Verification items for the finished model (mm, model axes). Face numbers are marked on the shaded views. A direction names the side the tool comes from. Give positions to 0.01 mm unless a question says otherwise; leave off trailing zeros. Write each loop counter-clockwise with the first axis right and the second up, starting at its lowest first coordinate (ties: lowest second). Pieces come first, ordered by that corner, then holes. Notation, with made-up numbers: M -5,35 L 21,35 A7 cw 21,43 Z; hole C -30.5,41.25 d10. An arc over 180 degrees is marked long. Write item = value, one per line.
from build123d import *

# Parameters (mm, degrees)
SKETCH_1_W          = 42
SKETCH_1_H          = 7
SKETCH_1_R          = 1.55
EXTRUDE_5_DEPTH     = 3
SKETCH_1_6_W        = 42
SKETCH_1_6_H        = 2
EXTRUDE_6_DEPTH     = 13
CUT_EXTRUDE_1_DEPTH = 13


with BuildPart() as part:
    # Sketch 1 → Extrude 5 (new body)
    with BuildSketch(Plane.XY):
        with Locations((26, 8.5)):
            Rectangle(SKETCH_1_W, SKETCH_1_H)
        with Locations((12, 8.4)):
            Circle(SKETCH_1_R, mode=Mode.SUBTRACT)
        with Locations((40, 8.4)):
            Circle(SKETCH_1_R, mode=Mode.SUBTRACT)
    extrude(amount=EXTRUDE_5_DEPTH)

    # Sketch 1_6 → Extrude 6 (add)
    with BuildSketch(Plane.XY):
        with Locations((26, 13)):
            Rectangle(SKETCH_1_6_W, SKETCH_1_6_H)
    extrude(amount=EXTRUDE_6_DEPTH)

    # Sketch 4 → Cut-Extrude 1 (cut)
    with BuildSketch(Plane(origin=(0, 14, 0), x_dir=(1, 0, 0), z_dir=(0, 1, 0))):
        with BuildLine():
            ThreePointArc((15, -6.45), (13.45, -8), (15, -9.55))
            Line((15, -9.55), (15, -6.45))
        make_face()
        with BuildLine():
            Line((15, -6.45), (15, -9.55))
            ThreePointArc((15, -9.55), (16.096015511, -9.096015511), (16.55, -8))
            ThreePointArc((16.55, -8), (16.096015511, -6.903984489), (15, -6.45))
        make_face()
        with BuildLine():
            ThreePointArc((37, -6.45), (35.45, -8), (37, -9.55))
            Line((37, -9.55), (37, -6.45))
        make_face()
        with BuildLine():
            Line((37, -6.45), (37, -9.55))
            ThreePointArc((37, -9.55), (38.096015511, -9.096015511), (38.55, -8))
            ThreePointArc((38.55, -8), (38.096015511, -6.903984489), (37, -6.45))
        make_face()
    extrude(amount=-CUT_EXTRUDE_1_DEPTH, mode=Mode.SUBTRACT)


solid = part.part
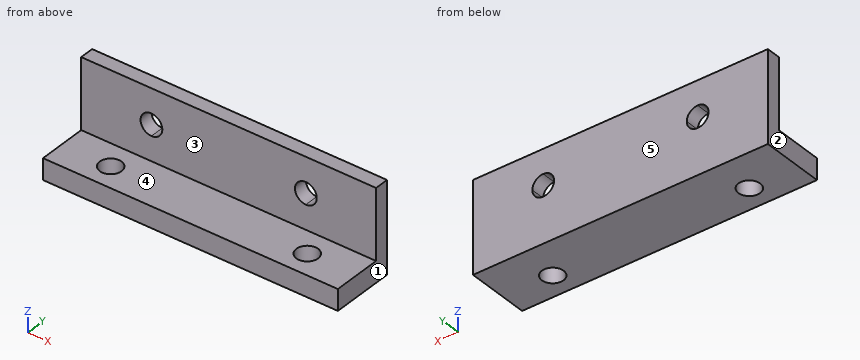
1) Depth check by flat-ended pin: P1, Ø3.5, axis at x = 32, y = 7, coming from the +Z side. Enter the tip coordinate at first touch or a pass-through.
From the geometry:
P1 = 3
2) Cross-section at D-D on x = 30.5. Record the boundary of the cut face in (y, z), plus the area to 3 significant figures.
From the geometry:
outline = M 5,0 L 14,0 L 14,13 L 12,13 L 12,3 L 5,3 Z
area = 47.0 mm^2
3) Tool access check on the marked faces 4 and 5. Record the directions out of +Z, -Z, +X, -X, +Y, -Y that give a thin tool (end or side, any length) a straight path to the whole face; none if there is none.
From the geometry:
face_4 = +Z, +X, -X, -Y
face_5 = +Z, -Z, +X, -X, +Y
4) Cross-section at B-B on y = 8.4. Record the boundary of the cut face in (x, z), plus the area to 3 significant figures.
From the geometry:
outline = M 5,0 L 10.45,0 L 10.45,3 L 5,3 Z; M 13.55,0 L 38.45,0 L 38.45,3 L 13.55,3 Z; M 41.55,0 L 47,0 L 47,3 L 41.55,3 Z
area = 107 mm^2
5) Material ranges on probe 1 along X at (y, z) = (8.5, 2.25); probe 2 along Y at (x, z) = (40, 1.3); probe 3 along Y at (x, z) = (37, 5.75), recorded low to high. Write a range as from..to.
From the geometry:
probe_1 = 5..10.45, 13.55..38.45, 41.55..47
probe_2 = 5..6.85, 9.95..14
probe_3 = 12..14
6) Draft check along X on the marked faces 1, 2 and 3. Enter one of: +X half, -X half, draft (parallel to the pull), parting line (faces both ways), or undercut.
From the geometry:
face_1 = +X half
face_2 = -X half
face_3 = draft
7) Cross-section at C-C on z = 1. Record the boundary of the cut face in (x, y).
From the geometry:
outline = M 5,5 L 47,5 L 47,14 L 5,14 Z; hole C 12,8.4 d3.1; hole C 40,8.4 d3.1
8) Cross-section at A-A on x = 12. Record the boundary of the cut face in (y, z).
From the geometry:
outline = M 5,0 L 6.85,0 L 6.85,3 L 5,3 Z; M 9.95,0 L 14,0 L 14,13 L 12,13 L 12,3 L 9.95,3 Z
